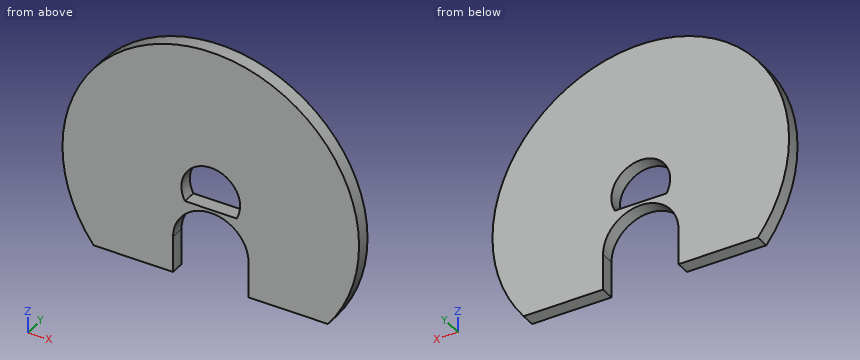
```python
from build123d import *

# Parameters (mm, degrees)
BOSS_EXTRUDE1_DEPTH = 6.35
CUT_EXTRUDE1_DEPTH  = 96.402278275


with BuildPart() as part:
    # Sketch2 → Boss-Extrude1 (new body)
    with BuildSketch(Plane(origin=(0, 0, 0), x_dir=(1, 0, 0), z_dir=(0, 1, 0))):
        with BuildLine():
            Line((-53.169638658, 41.275), (-17.145, 41.275))
            Line((-17.145, 41.275), (-17.145, 24.892))
            ThreePointArc((-17.145, 24.892), (0, 7.747), (17.145, 24.892))
            Line((17.145, 24.892), (17.145, 41.275))
            Line((17.145, 41.275), (53.169638658, 41.275))
            ThreePointArc((53.169638658, 41.275), (0, -67.31), (-53.169638658, 41.275))
        make_face()
    extrude(amount=BOSS_EXTRUDE1_DEPTH)

    # Sketch3 → Cut-Extrude1 (cut, through all)
    with BuildSketch(Plane(origin=(0, 6.35, 0), x_dir=(1, 0, 0), z_dir=(0, 1, 0))):
        with BuildLine():
            Line((-11.7475, 6.310187695), (11.7475, 6.310187695))
            ThreePointArc((11.7475, 6.310187695), (0, -13.335), (-11.7475, 6.310187695))
        make_face()
    extrude(amount=-CUT_EXTRUDE1_DEPTH, mode=Mode.SUBTRACT)


solid = part.part
```
Verification items for the finished model (mm, model axes). Round coordinates to 2 decimals unless told otherwise and drop trailing zeros. Write each loop counter-clockwise with the first axis right and the second up, starting at its lowest first coordinate (ties: lowest second). Pieces come first, ordered by that corner, then holes.
1. Gauge pin test, flat end, axial feed: P1, Ø3, axis at y = 4.5, z = -11.5, coming from the -X side. Record the tip position at first contact, or that the pin passes through.
2. Section check D-D on x = -24.5. Enter the section's corners in (y, z) (3 decimals).
3. Section check A-A on z = 0. Enter the section's corners in (x, y) (3 decimals), plus the area to 3 significant figures.
4. Scan lines: L1, parallel to X at y = 4.75, z = 0 (3 decimals); L2, parallel to X at y = 1.5, z = -34 (3 decimals); L3, parallel to Z at x = -2, y = 0.5. Record each from-to range of solid material in increasing order.
5. Section check C-C on y = 2.5. Enter the section's corners in (x, z) (1 decimal).
6. Section check B-B on x = 0. Enter the section's corners in (y, z) (3 decimals).
Answer:
1. P1: stops at x = -66.56
2. outline: (0, -41.275) - (6.35, -41.275) - (6.35, 62.693) - (0, 62.693) - close
3. outline: (-67.31, 0) - (-13.335, 0) - (-13.335, 6.35) - (-67.31, 6.35) - close; (13.335, 0) - (67.31, 0) - (67.31, 6.35) - (13.335, 6.35) - close
3. area: 685 mm2
4. L1: x = -67.31 to -13.335, 13.335 to 67.31
4. L2: x = -58.092 to -17.145, 17.145 to 58.092
4. L3: z = -7.86 to -6.31, 13.18 to 67.28
5. outline: (-53.2, -41.3) - (-17.1, -41.3) - (-17.1, -24.9) arc R17.1 cw to (17.1, -24.9) - (17.1, -41.3) - (53.2, -41.3) arc R67.3 ccw (long way) to start; hole (-11.7, -6.3) - (11.7, -6.3) arc R13.3 ccw (long way) to start
6. outline: (0, -7.747) - (6.35, -7.747) - (6.35, -6.31) - (0, -6.31) - close; (0, 13.335) - (6.35, 13.335) - (6.35, 67.31) - (0, 67.31) - close
